```python
from build123d import *

# Parameters (mm, degrees)
SKETCH1_R           = 5.85
BOSS_EXTRUDE1_DEPTH = 3.6
SKETCH3_R           = 2
CUT_EXTRUDE1_DEPTH  = 4


with BuildPart() as part:
    # Sketch1 → Boss-Extrude1 (new body)
    with BuildSketch(Plane(origin=(0, 0, 0), x_dir=(1, 0, 0), z_dir=(0, 1, 0))):
        with Locations(Location((0, 0, 0), (0, 0, 270))):
            Circle(SKETCH1_R)
    extrude(amount=BOSS_EXTRUDE1_DEPTH)

    # Sketch2 → Cut-Revolve1 (revolve, cut)
    with BuildSketch(Plane.XY):
        with BuildLine():
            Line((0, 1), (0, 11))
            ThreePointArc((0, 11), (5, 6), (0, 1))
        make_face()
    revolve(axis=Axis((0, 1, 0), (0, 1, 0)), mode=Mode.SUBTRACT)

    # Sketch3 → Cut-Extrude1 (cut)
    with BuildSketch(Plane.XZ):
        with Locations(Location((0, 0, 0), (0, 0, 270))):
            Circle(SKETCH3_R)
    extrude(amount=-CUT_EXTRUDE1_DEPTH, mode=Mode.SUBTRACT)


solid = part.part
```
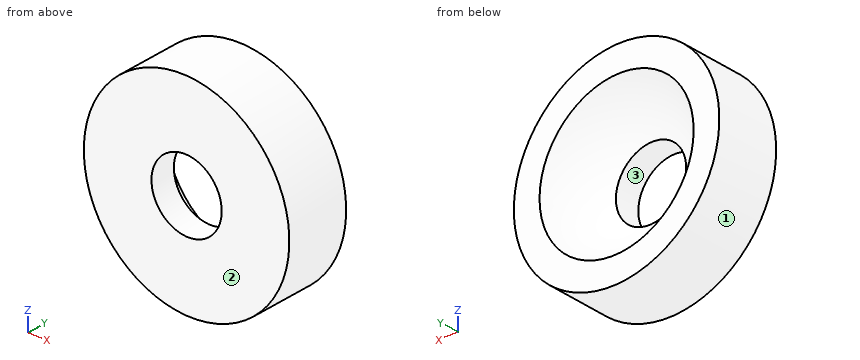
Work out the finished part from the listing and answer in its coordinate system (mm). Face numbers are marked on the shaded views. Give positions to 0.01 mm unless a question says otherwise; leave off trailing zeros. Order: outer loops, then holes, each group sorted by start corner. A loop starts at its lowest first (then second) coordinate and runs counter-clockwise, first axis right, second up.
1. Section D-D, the plane x = 3 is taken. Determine the outline of the cut face in (y, z).
Result sheet:
outline: (0, -5.02) - (3.6, -5.02) - (3.6, -3.2) arc R4 cw to (3.6, 3.2) - (3.6, 5.02) - (0, 5.02) - close
2. Section C-C, the plane y = 1.15 is taken. Determine the outline of the cut face in (x, z).
Result sheet:
outline: circle Ø11.7 at (0, 0); hole circle Ø4 at (0, 0)
3. Straight lines are drawn through the part: L1, parallel to X at y = 0.75, z = 0; L2, parallel to Z at x = -0.5, y = 3.3; L3, parallel to Z at x = 2, y = 3. For each, find the intervals that lie inside material, in ascending order.
Result sheet:
L1: x = -5.85 to -2, 2 to 5.85
L2: z = -5.83 to -4.18, 4.18 to 5.83
L3: z = -5.5 to -3.46, 3.46 to 5.5
4. Section B-B, the plane z = 0 is taken. Determine the outline of the cut face in (x, y), and give its area (3 significant figures).
Result sheet:
outline: (-5.85, 0) - (-2, 0) - (-2, 1.42) arc R5 cw to (-4.39, 3.6) - (-5.85, 3.6) - close; (2, 0) - (5.85, 0) - (5.85, 3.6) - (4.39, 3.6) arc R5 cw to (2, 1.42) - close
area: 21.3 mm2
5. The mould has two halves that part along X. Classify the marked faces 1, 2 and 3: released by +X, released by -X, zero draft, split by the parting line, or undercut.
Result sheet:
face 1: split by the parting line
face 2: zero draft
face 3: undercut
6. Each of these flat-tipped pins is pushed along its axis until it touches: P1, Ø1.5, axis at x = -3.5, z = 0.5, coming from the +Y side; P2, Ø1.5, axis at y = 2.5, z = -2, coming from the -X side; P3, Ø5, axis at x = -4, z = 0, coming from the -Y side; P4, Ø1, axis at x = 3.5, y = 2.5, coming from the -Z side. Where does it stop, or does it pass through?
Result sheet:
P1: stops at y = 3.42
P2: stops at x = -5.71
P3: stops at y = 0
P4: stops at z = -5.02
7. Section A-A, the plane x = 0 is taken. Determine the outline of the cut face in (y, z).
Result sheet:
outline: (0, -5.85) - (3.6, -5.85) - (3.6, -4.39) arc R5 cw to (1.42, -2) - (0, -2) - close; (0, 2) - (1.42, 2) arc R5 cw to (3.6, 4.39) - (3.6, 5.85) - (0, 5.85) - close
